Part model, mm, in its own coordinate system. Face numbers are marked on the shaded views. A direction names the side the tool comes from. Give positions to 0.01 mm unless a question says otherwise; leave off trailing zeros. Write each loop counter-clockwise with the first axis right and the second up, starting at its lowest first coordinate (ties: lowest second). Pieces come first, ordered by that corner, then holes.
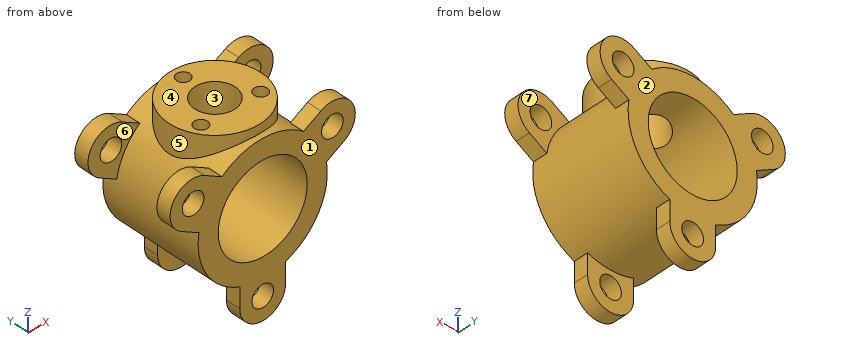
from build123d import *

# Parameters (mm, degrees)
SKETCH1_R               = 35.7124
SKETCH1_R_2             = 24.6126
BOSS_EXTRUDE1_DEPTH     = 57.15
SKETCH2_R               = 5.969
BOSS_EXTRUDE2_DEPTH     = 7.9502
CIRPATTERN1_COUNT       = 3
MIRROR1_COPY_1_SKETCH_R = 5.969
MIRROR1_COPY_1_DEPTH    = 7.9502
MIRROR1_COPY_2_SKETCH_R = 5.969
MIRROR1_COPY_2_DEPTH    = 7.9502
SKETCH3_R               = 25.4
BOSS_EXTRUDE3_DEPTH     = 19.05
CUT_EXTRUDE1_START      = -57.15
SKETCH4_R               = 24.6126
CUT_EXTRUDE1_DEPTH      = 57.15
SKETCH6_R               = 11.1125
CUT_EXTRUDE2_DEPTH      = 57.15
SKETCH7_R               = 3.636030774
CUT_EXTRUDE3_DEPTH      = 9.525


with BuildPart() as part:
    # Sketch1 → Boss-Extrude1 (new body)
    with BuildSketch(Plane(origin=(0, 0, 0), x_dir=(1, 0, 0), z_dir=(0, 1, 0))):
        with Locations(Location((0, 0, 0), (0, 0, 270))):
            Circle(SKETCH1_R)
        with Locations(Location((0, 0, 0), (0, 0, 270))):
            Circle(SKETCH1_R_2, mode=Mode.SUBTRACT)
    extrude(amount=BOSS_EXTRUDE1_DEPTH)

    # Sketch2 → Boss-Extrude2 (add)
    with BuildSketch(Plane(origin=(0, 57.15, 0), x_dir=(1, 0, 0), z_dir=(0, 1, 0))):
        with BuildLine():
            Line((-12.7, 44.45), (-12.7, 33.377919554))
            Line((-12.7, 33.377919554), (12.7, 33.377919554))
            Line((12.7, 33.377919554), (12.7, 44.45))
            ThreePointArc((12.7, 44.45), (0, 57.15), (-12.7, 44.45))
        make_face()
        with Locations(Location((0, 44.45, 0), (0, 0, 270))):
            Circle(SKETCH2_R, mode=Mode.SUBTRACT)
    boss_extrude2 = extrude(amount=-BOSS_EXTRUDE2_DEPTH)

    # CirPattern1: Boss-Extrude2 ×3 about axis
    cirpattern1_axis = Axis((0, 0, 0), (0, 1, 0))
    for i in range(1, CIRPATTERN1_COUNT):
        add(boss_extrude2.rotate(cirpattern1_axis, i * 360 / CIRPATTERN1_COUNT))

    # Mirror1: Boss-Extrude2 across plane
    add(boss_extrude2.mirror(Plane.ZX.offset(28.575)))

    # Mirror1 copy 1 sketch → Mirror1 copy 1 (add)
    with BuildSketch(Plane(origin=(0, 0, 0), x_dir=(-0.4999999999999998, 0, -0.8660254037844387), z_dir=(0, -1, 0))):
        with BuildLine():
            Line((-12.7, -44.45), (-12.7, -33.377919554))
            Line((-12.7, -33.377919554), (12.7, -33.377919554))
            Line((12.7, -33.377919554), (12.7, -44.45))
            ThreePointArc((12.7, -44.45), (0, -57.15), (-12.7, -44.45))
        make_face()
        with Locations((0, -44.45)):
            Circle(MIRROR1_COPY_1_SKETCH_R, mode=Mode.SUBTRACT)
    extrude(amount=-MIRROR1_COPY_1_DEPTH)

    # Mirror1 copy 2 sketch → Mirror1 copy 2 (add)
    with BuildSketch(Plane(origin=(0, 0, 0), x_dir=(-0.5000000000000004, 0, 0.8660254037844384), z_dir=(0, -1, 0))):
        with BuildLine():
            Line((-12.7, -44.45), (-12.7, -33.377919554))
            Line((-12.7, -33.377919554), (12.7, -33.377919554))
            Line((12.7, -33.377919554), (12.7, -44.45))
            ThreePointArc((12.7, -44.45), (0, -57.15), (-12.7, -44.45))
        make_face()
        with Locations((0, -44.45)):
            Circle(MIRROR1_COPY_2_SKETCH_R, mode=Mode.SUBTRACT)
    extrude(amount=-MIRROR1_COPY_2_DEPTH)

    # Sketch3 → Boss-Extrude3 (add)
    with BuildSketch(Plane.XY.offset(40.4876)):
        with Locations((-0.044379285, 28.575)):
            Circle(SKETCH3_R)
    extrude(amount=-BOSS_EXTRUDE3_DEPTH)

    # Sketch4 → Cut-Extrude1 (cut)
    with BuildSketch(Plane(origin=(0, 57.15, 0), x_dir=(1, 0, 0), z_dir=(0, 1, 0)).offset(CUT_EXTRUDE1_START)):
        with Locations(Location((0, 0, 0), (0, 0, 270))):
            Circle(SKETCH4_R)
    extrude(amount=CUT_EXTRUDE1_DEPTH, mode=Mode.SUBTRACT)

    # Sketch6 → Cut-Extrude2 (cut)
    with BuildSketch(Plane.XY.offset(40.4876)):
        with Locations((-0.044379285, 28.575)):
            Circle(SKETCH6_R)
    extrude(amount=-CUT_EXTRUDE2_DEPTH, mode=Mode.SUBTRACT)

    # Sketch7 → Cut-Extrude3 (cut)
    with BuildSketch(Plane.XY.offset(40.4876)):
        with Locations((0, 47.625)):
            Circle(SKETCH7_R)
        with Locations((16.431215014, 19.011566412)):
            Circle(SKETCH7_R)
        with Locations((-16.56435287, 19.088433588)):
            Circle(SKETCH7_R)
    extrude(amount=-CUT_EXTRUDE3_DEPTH, mode=Mode.SUBTRACT)


solid = part.part
1) Flat gauge pins, fed straight in: P1, Ø12, axis at y = 50, z = -28.5, coming from the -X side; P2, Ø2.5, axis at y = 52.5, z = -36.5, coming from the +X side; P3, Ø1.5, axis at x = -37.5, y = 28, coming from the +Z side; P4, Ø2, axis at y = 51, z = -17.5, coming from the +X side. Where does each tip first touch, or does it go through?
Check result:
P1: stops at x = -27.73
P2: stops at x = 12.7
P3: passes through
P4: stops at x = 31.67
2) 3-axis set-ups, long thin cutter, end or side, ignore diameter. For the marked faces 5, 6 and 7: which of +Z, -Z, +X, -X, +Y, -Y reach the whole face in a straight line?
Check result:
face 5: +Z
face 6: +Z, -X
face 7: +Z, +X
3) Saw through at A-A (z = 0). Write the cut outline in (x, y), and give its area (3 significant figures).
Check result:
outline: (-35.71, 0) - (-24.61, 0) - (-24.61, 57.15) - (-35.71, 57.15) - close; (24.61, 0) - (35.71, 0) - (35.71, 57.15) - (24.61, 57.15) - close
area: 1,270 mm2
4) Saw through at B-B (x = 0). State how many separate pieces and enclosed holes the cut face has, and give its area (3 significant figures).
Check result:
separate pieces: 5
enclosed holes: 0
area: 1,240 mm2
5) Mould opens along Y. For the marked faces 1, 2, 3 and 4 say: +Y half, -Y half, draft (parallel to the pull), parting line (faces both ways), or undercut.
Check result:
face 1: -Y half
face 2: +Y half
face 3: undercut
face 4: draft
6) Saw through at D-D (x = -15.5). Write the cut outline in (y, z).
Check result:
outline: (0, -32.17) - (57.15, -32.17) - (57.15, -19.12) - (0, -19.12) - close; (0, 19.12) - (57.15, 19.12) - (57.15, 32.17) - (48.73, 32.17) - (48.73, 40.49) - (22.57, 40.49) - (22.57, 30.96) - (15.61, 30.96) - (15.61, 40.49) - (8.42, 40.49) - (8.42, 32.17) - (0, 32.17) - close
7) Saw through at C-C (y = 38). Write the cut outline in (x, z), and give its area (3 significant figures).
Check result:
outline: (-23.63, 26.78) arc R35.71 ccw (long way) to (23.54, 26.85) - (23.54, 40.49) - (5.84, 40.49) - (5.84, 23.91) arc R24.61 cw (long way) to (-5.93, 23.89) - (-5.93, 40.49) - (-23.63, 40.49) - close
area: 2,270 mm2
8) Drill centre lines: L1, parallel to Y at x = 0, z = 37; L2, parallel to Y at x = -37, z = 9; L3, parallel to X at y = 51, z = -44. Where is each one in solid material? Low to high.
Check result:
L1: y = 3.18 to 17.46, 39.69 to 43.99, 51.26 to 53.97
L2: y = 0 to 7.95, 49.2 to 57.15
L3: x = -12.7 to -5.95, 5.95 to 12.7
